Autodesk Inventor part; units mm, degrees
ref_plane "YZ Plane" through (0, 0, 0) normal (1, 0, 0) x (0, 1, 0)
ref_plane "XZ Plane" through (0, 0, 0) normal (0, 1, 0) x (-1, 0, 0)
ref_plane "XY Plane" through (0, 0, 0) normal (0, 0, 1) x (1, 0, 0)
sketch "Sketch1" plane through (0, 0, 0) normal (1, 0, 0) x (0, 1, 0)
  line L0 (-11, 11) -> (11, 11)
  line L1 (11, 11) -> (11, -11)
  line L2 (11, -11) -> (-11, -11)
  line L3 (-11, -11) -> (-11, 11)
  point P0 (0, 0)
  dimension "d0" = 22
  dimension "d1" = 22
  dimension "d2" = 11
  dimension "d3" = 11
extrude "Extrusion1" add sketch "Sketch1" along normal blind 0.8
sketch "Sketch2" plane through (0.8, 0, 0) normal (1, 0, 0) x (0, 0, -1)
  circle A0 centre (0, -8.5) radius 1.25
  circle A1 centre (0, 8.5) radius 1.25
  point P0 (0, 0)
  dimension "d6" = 2.5
  dimension "d7" = 2.5
  dimension "d8" = 8.5
  dimension "d9" = 8.5
extrude "Extrusion2" cut sketch "Sketch2" against normal blind 10
properties part number "PCB"
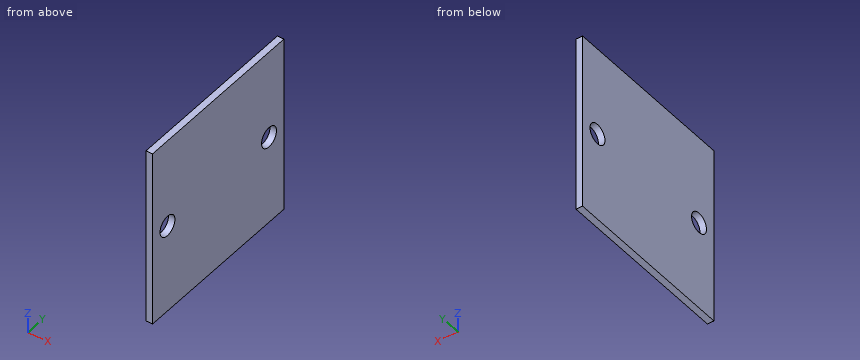
Geometry check sheet. Reference: the model listing, model coordinates, mm. Coordinates: 2 decimals unless noted, no trailing zeros. Order: outer loops, then holes, each group sorted by start corner. A loop starts at its lowest first (then second) coordinate and runs counter-clockwise, first axis right, second up. Notation, with made-up numbers: (50, 66) - (91, 66) arc R22 cw to (91, 75) - close; hole circle Ø1 at (82.25, 80.25). An arc over 180 degrees is marked (long way). One line per item, written item: value.
(1) Sectioned sample at B-B (y = 8.5). Enter the section's corners in (x, z), and give its area (3 significant figures).
Data:
outline: (0, -11) - (0.8, -11) - (0.8, -1.25) - (0, -1.25) - close; (0, 1.25) - (0.8, 1.25) - (0.8, 11) - (0, 11) - close
area: 15.6 mm^2
(2) Depth check by flat-ended pin: pin 1 Ø2 at (y, z) = (-8.5, 0) entering from -X. Enter the tip coordinate at first touch or a pass-through.
Data:
pin 1: passes through
(3) Thickness scan on probe 1 along Y at (x, z) = (0.6, 0); probe 2 along Y at (x, z) = (0.4, -0.5). Record the ranges inside material, lowest first. Write a range as from..to.
Data:
probe 1: y = -11..-9.75, -7.25..7.25, 9.75..11
probe 2: y = -11..-9.65, -7.35..7.35, 9.65..11
(4) Sectioned sample at C-C (x = 0.45). Enter the section's corners in (y, z).
Data:
outline: (-11, -11) - (11, -11) - (11, 11) - (-11, 11) - close; hole circle Ø2.5 at (-8.5, 0); hole circle Ø2.5 at (8.5, 0)
(5) Sectioned sample at A-A (z = 0). Enter the section's corners in (x, y), and give its area (3 significant figures).
Data:
outline: (0, -11) - (0.8, -11) - (0.8, -9.75) - (0, -9.75) - close; (0, -7.25) - (0.8, -7.25) - (0.8, 7.25) - (0, 7.25) - close; (0, 9.75) - (0.8, 9.75) - (0.8, 11) - (0, 11) - close
area: 13.6 mm^2
